Model file for the job. Use its own axes, mm. Face numbers are marked on the shaded views. A direction names the side the tool comes from. Give positions to 0.01 mm unless a question says otherwise; leave off trailing zeros. Order: outer loops, then holes, each group sorted by start corner. A loop starts at its lowest first (then second) coordinate and runs counter-clockwise, first axis right, second up. Notation, with made-up numbers: (33.25, 77.25) - (69.25, 77.25) arc R23 ccw to (69.25, 109.25) - close; hole circle Ø2 at (82, 38). An arc over 180 degrees is marked (long way). Use CSV: the item, a comma, the result in double quotes. Start each with the question number.
(1) Probe L1, parallel to X at y = 9, z = -3; L2, parallel to X at y = -0.5, z = 38; L3, parallel to Z at x = -18, y = -33.5. List the from-to ranges inside material, lowest first.
(2) Pull direction X, two halves, no side cores. Call the marked faces 1, 2 and 3: +X half, -X half, draft (parallel to the pull), parting line (faces both ways), or undercut.
(3) Band-saw the part on B-B, the plane x = 56. Give the cut face in (y, z).
(4) Band-saw the part on C-C, the plane z = 34. Give the cut face in (x, y), then the cut area to 3 significant figures.
(5) Tool access for the marked faces 4, 5 and 6: list every direction of +Z, -Z, +X, -X, +Y, -Y with a clear straight run to the whole face (end or side of a thin tool).
(6) Drop flat-ended pins along their axis: pin 1 Ø4 at (x, y) = (77.5, -7) entering from +Z; pin 2 Ø3 at (y, z) = (-22, 38.5) entering from -X; pin 3 Ø1.8 at (y, z) = (-4, -4) entering from -X; pin 4 Ø3 at (y, z) = (-0.5, 6.5) entering from +X. Give the stop position or say it passes through.
(7) Band-saw the part on A-A, the plane y = 3. Give the cut face in (x, z), then the cut area to 3 significant figures.
from build123d import *

# Parameters (mm, degrees)
F0_W     = 146
F0_H     = 91
F1_DEPTH = 55
F3_DEPTH = 91


with BuildPart() as f1:
    # F0 (on Top) → F1 (new body)
    with BuildSketch(Plane.XY):
        Rectangle(F0_W, F0_H)
    extrude(amount=F1_DEPTH)

    # F2 (on face) → F3 (join, through all)
    with BuildSketch(Plane.XZ.offset(45.5)):
        Polygon((-72, 0), (-73, 0), (-73, -4.85), (-85.75, -4.85), (-85.75, -5.85), (-73, -5.85), (-72, -5.85), align=None)
        Polygon((73, -4.85), (73, 0), (72, 0), (72, -5.85), (73, -5.85), (85.75, -5.85), (85.75, -4.85), align=None)
    extrude(amount=-F3_DEPTH)


solid = f1.part
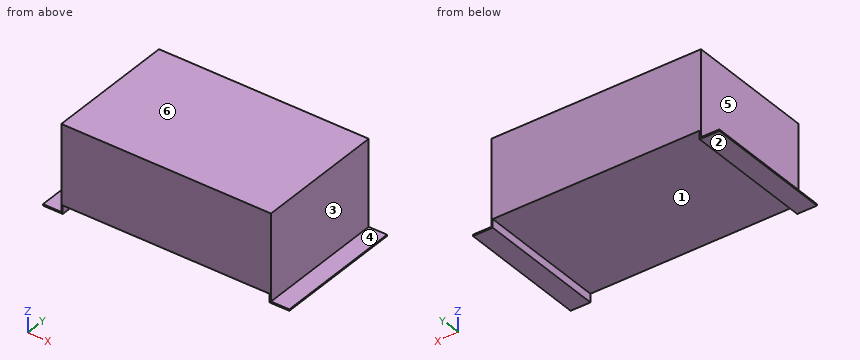
Answer block:
1,L1,"x = -73 to -72, 72 to 73"
1,L2,"x = -73 to 73"
1,L3,"z = 0 to 55"
2,face 1,"undercut"
2,face 2,"draft"
2,face 3,"+X half"
3,outline,"(-45.5, 0) - (45.5, 0) - (45.5, 55) - (-45.5, 55) - close"
4,outline,"(-73, -45.5) - (73, -45.5) - (73, 45.5) - (-73, 45.5) - close"
4,area,"13,300 mm2"
5,face 4,"+Z, +X, +Y, -Y"
5,face 5,"+Z, -X, +Y, -Y"
5,face 6,"+Z, +X, -X, +Y, -Y"
6,pin 1,"stops at z = -4.85"
6,pin 2,"stops at x = -73"
6,pin 3,"stops at x = -85.75"
6,pin 4,"stops at x = 73"
7,outline,"(-85.75, -5.85) - (-72, -5.85) - (-72, 0) - (72, 0) - (72, -5.85) - (85.75, -5.85) - (85.75, -4.85) - (73, -4.85) - (73, 55) - (-73, 55) - (-73, -4.85) - (-85.75, -4.85) - close"
7,area,"8,070 mm2"
